Work out the finished part from the listing and answer in its coordinate system (mm). Face numbers are marked on the shaded views. A direction names the side the tool comes from. Coordinates: 2 decimals unless noted, no trailing zeros. Write each loop counter-clockwise with the first axis right and the second up, starting at its lowest first coordinate (ties: lowest second). Pieces come first, ordered by that corner, then holes. Notation, with made-up numbers: (-39.75, -2.75) - (5.25, -2.75) arc R21 cw to (5.25, 34.25) - close; hole circle Ø7 at (56.25, -21.75). An arc over 180 degrees is marked (long way). Use a Markdown table: item, result. Add a question column.
(1) For a pull along Y with two mould halves and no side action, classify the marked faces 4, 5 and 6 as released by +Y, released by -Y, zero draft, split by the parting line, or undercut.
(2) A tool of negligible diameter and unlimited length cuts with its end or side. For the marked faces 1, 2 and 3, from which of +Z, -Z, +X, -X, +Y, -Y can it reach the whole face along a straight path? Write none if from no direction.
(3) The part is cut by section C-C, the plane x = -9.5. Give the vertices of the cut face in (y, z).
(4) The part is cut by section D-D, the plane z = -12. Give the vertices of the cut face in (x, y).
(5) The part is cut by section A-A, the plane z = 0. Give the vertices of the cut face in (x, y), then the cut area to 3 significant figures.
(6) Find the intervals of material crossed by line 1 (Y direction, x = -5, z = 0); line 2 (Y direction, x = -4, z = 0); line 3 (X direction, y = -11, z = 4), in increasing order. Write a range as from..to.
(7) Given pin 1 Ø1.5 at (x, y) = (-4.5, 12.5) entering from +Z; pin 2 Ø1.5 at (x, z) = (-9.5, 4) entering from -Y; pin 3 Ø1 at (y, z) = (10, -7.5) entering from +X, each flat-ended and moving along its own axis, determine where each tip first touches the part or whether it passes through.
from build123d import *

# Parameters (mm, degrees)
SKETCH1_W           = 4.87911158
SKETCH1_H           = 4.7625
SKETCH2_R           = 4.25
BOSS_EXTRUDE1_DEPTH = 5.08


with BuildPart() as part:
    # Sketch1 → Revolve1 (revolve)
    with BuildSketch(Plane.XY, mode=Mode.PRIVATE) as revolve1_sk:
        with Locations((-2.43955579, 3.96875)):
            Rectangle(SKETCH1_W, SKETCH1_H)
        Polygon((-8.187387237, 1.5875), (-4.87911158, 1.5875), (-4.87911158, 6.35), (-4.87911158, 20.5), (-8.187387237, 20.5), align=None)
    revolve(revolve1_sk.sketch.rotate(Axis((0, 0, 0), (-1, 0, 0)), 90), axis=Axis((0, 0, 0), (-1, 0, 0)))

    # Sketch2 → Boss-Extrude1 (add)
    with BuildSketch(Plane.ZY.offset(8.187387237)):
        with Locations(Location((0, 12.6, 0), (0, 0, 180))):
            Circle(SKETCH2_R)
        with Locations(Location((12.6, 0, 0), (0, 0, 180))):
            Circle(SKETCH2_R)
        with Locations(Location((0, -12.6, 0), (0, 0, 180))):
            Circle(SKETCH2_R)
        with Locations(Location((-12.6, 0, 0), (0, 0, 180))):
            Circle(SKETCH2_R)
    extrude(amount=BOSS_EXTRUDE1_DEPTH)


solid = part.part
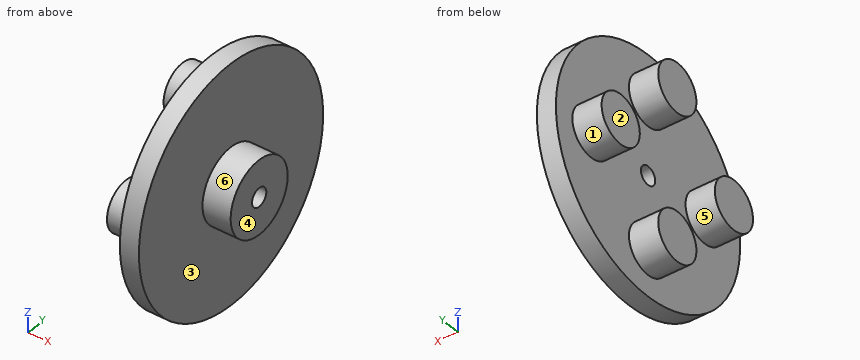
Model answer:
| question | item | result |
|---|---|---|
| 1 | face 4 | zero draft |
| 1 | face 5 | undercut |
| 1 | face 6 | split by the parting line |
| 2 | face 1 | -X |
| 2 | face 2 | +Z, -Z, -X, +Y, -Y |
| 2 | face 3 | +X |
| 3 | outline | circle Ø8.5 at (-12.6, 0); circle Ø8.5 at (0, -12.6); circle Ø8.5 at (0, 12.6); circle Ø8.5 at (12.6, 0) |
| 4 | outline | (-13.27, -4.21) - (-8.19, -4.21) - (-8.19, -16.62) - (-4.88, -16.62) - (-4.88, 16.62) - (-8.19, 16.62) - (-8.19, 4.21) - (-13.27, 4.21) - close |
| 5 | outline | (-13.27, -16.85) - (-8.19, -16.85) - (-8.19, -20.5) - (-4.88, -20.5) - (-4.88, -6.35) - (0, -6.35) - (0, -1.59) - (-8.19, -1.59) - (-8.19, -8.35) - (-13.27, -8.35) - close; (-13.27, 8.35) - (-8.19, 8.35) - (-8.19, 1.59) - (0, 1.59) - (0, 6.35) - (-4.88, 6.35) - (-4.88, 20.5) - (-8.19, 20.5) - (-8.19, 16.85) - (-13.27, 16.85) - close |
| 5 | area | 258 mm^2 |
| 6 | line 1 | -20.5..-1.59, 1.59..20.5 |
| 6 | line 2 | -6.35..-1.59, 1.59..6.35 |
| 6 | line 3 | -8.19..-4.88 |
| 7 | pin 1 | z = 16.73 |
| 7 | pin 2 | y = -15.34 |
| 7 | pin 3 | x = -4.88 |
